For this review, take the finished solid that the model builds, in its own axes (mm). A direction names the side the tool comes from. Round coordinates to 2 decimals unless told otherwise and drop trailing zeros. Write each loop counter-clockwise with the first axis right and the second up, starting at its lowest first coordinate (ties: lowest second). Pieces come first, ordered by that corner, then holes. Notation, with made-up numbers: (47, 35) -> (69, 35) arc R14 ccw to (69, 59) -> close; hole circle Ø1 at (47.25, 65.5). An arc over 180 degrees is marked (long way). Answer in a Markdown table with one row per item.
from build123d import *

# Parameters (mm, degrees)
F0_R     = 250
F1_DEPTH = 600
F2_W     = 20
F2_H     = 450
F3_DEPTH = 300


with BuildPart() as f1:
    # F0 (on Top) → F1 (new body)
    with BuildSketch(Plane.XY):
        with Locations((0, -15.917291)):
            Circle(F0_R)
    extrude(amount=F1_DEPTH)

    # F2 (on Front) → F3 (join)
    with BuildSketch(Plane.XZ):
        with Locations((55, 375)):
            Rectangle(F2_W, F2_H)
        with Locations((-55, 375)):
            Rectangle(F2_W, F2_H)
    extrude(amount=F3_DEPTH)


solid = f1.part
1) Consider section C-C on x = 0. State the section outline as (y, z) points.
Solved:
| item | result |
|---|---|
| outline | (-265.92, 0) -> (234.08, 0) -> (234.08, 600) -> (-265.92, 600) -> close |
2) For line 1 (X direction, y = -17.5, z = 195) (3 decimals); line 2 (Y direction, x = 9, z = 307.5); line 3 (X direction, y = 92, z = 331.5), list the stretches that pass through material, from the lowest coordinate up. Write a range as [from, to].
Solved:
| item | result |
|---|---|
| line 1 | [-249.995, 249.995] |
| line 2 | [-265.76, 233.92] |
| line 3 | [-225.51, 225.51] |
3) Consider section B-B on y = -93. State the section outline as (x, z) points, then the cut area to 3 significant figures.
Solved:
| item | result |
|---|---|
| outline | (-237.82, 0) -> (237.82, 0) -> (237.82, 600) -> (-237.82, 600) -> close |
| area | 285,000 mm² |
4) Consider section A-A on z = 238. State the section outline as (x, y) points.
Solved:
| item | result |
|---|---|
| outline | (-65, -300) -> (-45, -300) -> (-45, -261.83) arc R250 ccw to (45, -261.83) -> (45, -300) -> (65, -300) -> (65, -257.32) arc R250 ccw (long way) to (-65, -257.32) -> close |
5) For faces 4 (the flat face through (-45, -281, 372)), 5 (the flat face through (55, -278, 150)), 6 (the flat face through (-55, -278, 150)), 7 (the flat face through (65, -278, 372)), list the 3-axis set-ups (+Z, -Z, +X, -X, +Y, -Y) from which the entire face can be reached by the end or side of a thin tool; tool diameter is ignored.
Solved:
| item | result |
|---|---|
| face 4 | +Z, -Z, -Y |
| face 5 | -Z, +X, -Y |
| face 6 | -Z, -X, -Y |
| face 7 | +Z, -Z, +X, -Y |
6) Mouldability with a two-part tool opening along X and no side actions: class faces 1 (the flat face through (-3, -12, 0)), 2 (the flat face through (45, -281, 372)), 3 (the flat face through (-65, -278, 372)) as pulls with the +X half, pulls with the -X half, needs draft (parallel to the pull), parting line crosses it, or undercut.
Solved:
| item | result |
|---|---|
| face 1 | needs draft |
| face 2 | undercut |
| face 3 | pulls with the -X half |
7) Clearance check with flat-ended pins moving along their axes: pin 1 Ø10 at (x, y) = (-51, -272) entering from -Z; pin 2 Ø2 at (y, z) = (-173, 107) entering from -X; pin 3 Ø1.5 at (x, z) = (67.5, 466.5) entering from +Y. State where each tip first meets the part, or that it passes through.
Solved:
| item | result |
|---|---|
| pin 1 | z = 150 |
| pin 2 | x = -195.29 |
| pin 3 | y = 225.01 |
